Design review of the part built by this model. Coordinates are the model's own, in mm. A direction names the side the tool comes from. Coordinates: 2 decimals unless noted, no trailing zeros. Loops run counter-clockwise (first coordinate to the right, second up) from the corner with the lowest first, then second, coordinate; pieces in that order, holes last. Notation, with made-up numbers: (-7, 10.5) -> (4, 10.5) arc R29 cw to (4, 46.5) -> close; hole circle Ø5 at (-15, 3). An arc over 180 degrees is marked (long way). Use CSV: the item, a comma, the result in double quotes.
```python
from build123d import *

# Parameters (mm, degrees)
BOSS_EXTRUDE1_DEPTH = 279.4
SKETCH2_R           = 3.5
CUT_EXTRUDE1_DEPTH  = 27.9875
SKETCH3_R           = 3.175
CUT_EXTRUDE2_DEPTH  = 32.75


with BuildPart() as part:
    # Sketch1 → Boss-Extrude1 (new body, symmetric)
    with BuildSketch(Plane.XY):
        Polygon((-25.4, 31.75), (-25.4, 28.575), (-1.5875, 28.575), (-1.5875, 0), (1.5875, 0), (1.5875, 28.575), (25.4, 28.575), (25.4, 31.75), align=None)
    extrude(amount=BOSS_EXTRUDE1_DEPTH, both=True)

    # Sketch2 → Cut-Extrude1 (cut, through all)
    with BuildSketch(Plane(origin=(1.5875, 0, 0), x_dir=(0, 0, -1), z_dir=(1, 0, 0))):
        with Locations((-254, 15.875)):
            Circle(SKETCH2_R)
        with Locations((254, 15.875)):
            Circle(SKETCH2_R)
    extrude(amount=-CUT_EXTRUDE1_DEPTH, mode=Mode.SUBTRACT)

    # Sketch3 → Cut-Extrude2 (cut, through all)
    with BuildSketch(Plane(origin=(0, 31.75, 0), x_dir=(1, 0, 0), z_dir=(0, 1, 0))):
        with Locations((-12.7, 228.6)):
            Circle(SKETCH3_R)
        with Locations((12.7, 228.6)):
            Circle(SKETCH3_R)
        with Locations((12.7, -228.6)):
            Circle(SKETCH3_R)
        with Locations((-12.7, -228.6)):
            Circle(SKETCH3_R)
    extrude(amount=-CUT_EXTRUDE2_DEPTH, mode=Mode.SUBTRACT)


solid = part.part
```
Item 1: Clearance check with flat-ended pins moving along their axes: pin 1 (6 mm diameter, centred on x = 5, z = 86.5, fed in from -Y) (3 decimals); pin 2 (8.5 mm diameter, centred on y = 13, z = -5.5, fed in from -X); pin 3 (6 mm diameter, centred on y = 12, z = -87.5, fed in from +X). State where each tip first meets the part, or that it passes through.
Checked values:
pin 1,"y = 28.575"
pin 2,"x = -1.59"
pin 3,"x = 1.59"
Item 2: Machinability: for faces 1 (the face through (-1.588, 14, 4)), 2 (the face through (0, 27, 279.4)), 3 (the face through (13, 28.575, 4)), which of the approach directions +Z, -Z, +X, -X, +Y, -Y give a long, thin tool a straight path to every point of the face, cutting with its end or side? Answer none if there is none.
Checked values:
face 1,"+Z, -Z, -X, -Y"
face 2,"+Z, +X, -X, +Y, -Y"
face 3,"+Z, -Z, +X, -Y"
Item 3: To check wall thickness, follow line 1 along X through (y, z) = (29, -228); line 2 along Z through (x, y) = (12, 30); line 3 along X through (y, z) = (30.2, -228.6) (3 decimals). State the ranges of each line that lie inside material, in increasing order.
Checked values:
line 1,"-25.4 to -15.82, -9.58 to 9.58, 15.82 to 25.4"
line 2,"-279.4 to -231.7, -225.5 to 225.5, 231.7 to 279.4"
line 3,"-25.4 to -15.875, -9.525 to 9.525, 15.875 to 25.4"
Item 4: Add section B-B (y = 5). Give the boundary of the cut face in (x, z), then the cut area to 3 significant figures.
Checked values:
outline,"(-1.59, -279.4) -> (1.59, -279.4) -> (1.59, 279.4) -> (-1.59, 279.4) -> close"
area,"1,770 mm^2"
